Geometry check sheet. Reference: drawing and pictorial views, mm from the part's lowest x, y, z. Coordinates: 2 decimals unless noted, no trailing zeros. Loops run counter-clockwise (first coordinate to the right, second up) from the corner with the lowest first, then second, coordinate; pieces in that order, holes last. Notation, with made-up numbers: (41, 0) - (51, 0) arc R14 cw to (51, 12) - close; hole circle Ø4 at (64.25, -19.75). An arc over 180 degrees is marked (long way). One line per item, written item: value.
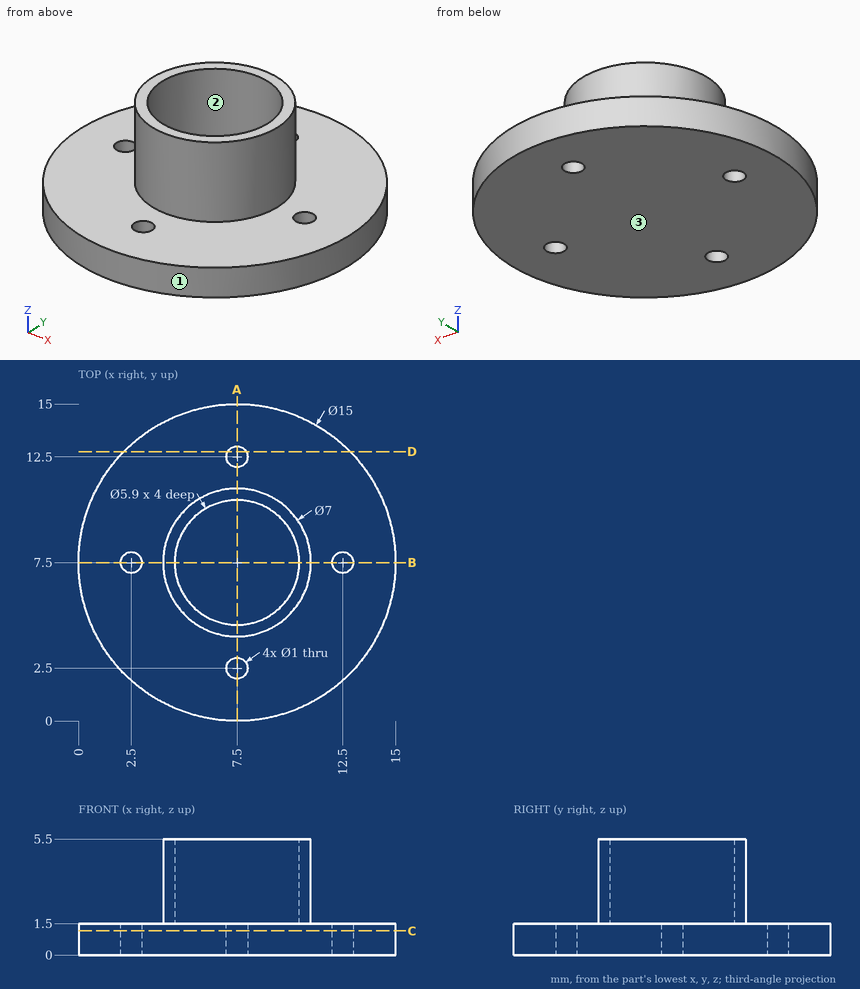
(1) Release check for a two-part mould opening along Y. For the marked faces 1, 2 and 3 record: pulls with the +Y half, pulls with the -Y half, needs draft (parallel to the pull), parting line crosses it, or undercut.
Reply:
face 1: parting line crosses it
face 2: undercut
face 3: needs draft
(2) Go/stop test with flat-tipped pins: pin 1 Ø7 at (x, y) = (7.5, 7.5) entering from -Z; pin 2 Ø1 at (x, y) = (2, 10.5) entering from +Z; pin 3 Ø2 at (y, z) = (3.5, 3.5) entering from +X. Record where each tip stops, or that it passes through.
Reply:
pin 1: z = 0
pin 2: z = 1.5
pin 3: x = 9.3
(3) Cross-section at C-C on z = 1.15. Record the cut outline in (x, y).
Reply:
outline: circle Ø15 at (7.5, 7.5); hole circle Ø1 at (2.5, 7.5); hole circle Ø1 at (7.5, 2.5); hole circle Ø1 at (7.5, 12.5); hole circle Ø1 at (12.5, 7.5)
(4) Material ranges on probe 1 along Y at (x, z) = (7.5, 0.4); probe 2 along Y at (x, z) = (7.5, 4.7); probe 3 along Z at (x, y) = (9.5, 14), recorded low to high. Write a range as from..to.
Reply:
probe 1: 0..2, 3..12, 13..15
probe 2: 4..4.55, 10.45..11
probe 3: 0..1.5
(5) Cross-section at D-D on y = 12.75. Record the cut outline in (x, z), and give its area (3 significant figures).
Reply:
outline: (2.14, 0) - (7.07, 0) - (7.07, 1.5) - (2.14, 1.5) - close; (7.93, 0) - (12.86, 0) - (12.86, 1.5) - (7.93, 1.5) - close
area: 14.8 mm2
(6) Cross-section at A-A on x = 7.5. Record the cut outline in (y, z).
Reply:
outline: (0, 0) - (2, 0) - (2, 1.5) - (0, 1.5) - close; (3, 0) - (12, 0) - (12, 1.5) - (11, 1.5) - (11, 5.5) - (10.45, 5.5) - (10.45, 1.5) - (4.55, 1.5) - (4.55, 5.5) - (4, 5.5) - (4, 1.5) - (3, 1.5) - close; (13, 0) - (15, 0) - (15, 1.5) - (13, 1.5) - close
